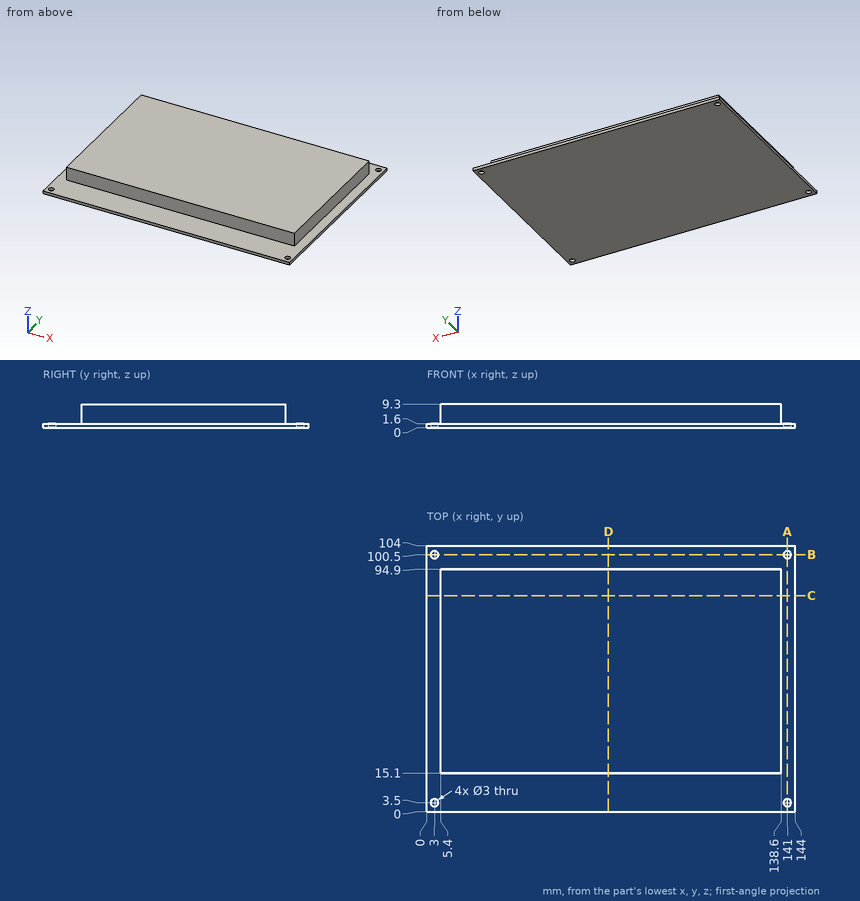
Geometry check sheet. Reference: drawing and pictorial views, mm from the part's lowest x, y, z. Round coordinates to 2 decimals unless told otherwise and drop trailing zeros. Loops run counter-clockwise (first coordinate to the right, second up) from the corner with the lowest first, then second, coordinate; pieces in that order, holes last. Notation, with made-up numbers: (6, 16) - (16, 16) arc R6 ccw to (16, 21) - close; hole circle Ø11 at (36, -31.75). An arc over 180 degrees is marked (long way). One line per question, with ' | ' between items. Start each with the question number.
1. Cross-section at A-A on x = 141. Record the cut outline in (y, z), then the cut area to 3 significant figures.
2. Depth check by flat-ended pin: pin 1 (2.5 mm diameter, centred on y = 43, z = 6, fed in from +X); pin 2 (4 mm diameter, centred on y = 47.5, z = 5.5, fed in from -X); pin 3 (5 mm diameter, centred on x = 141, y = 3.5, fed in from +Z). Enter the tip coordinate at first touch or a pass-through.
3. Cross-section at C-C on y = 84.5. Record the cut outline in (x, z).
4. Cross-section at B-B on y = 100.5. Record the cut outline in (x, z), then the cut area to 3 significant figures.
5. Scan lines: line 1 (X direction, y = 100.5, z = 0.8); line 2 (Y direction, x = 3, z = 1.1); line 3 (Z direction, x = 54, y = 10). Record each from-to range of solid material in increasing order. Write a range as [from, to].
6. Cross-section at D-D on x = 71. Record the cut outline in (y, z), then the cut area to 3 significant figures.
Taken from the geometry:
1) outline: (0, 0) - (2, 0) - (2, 1.6) - (0, 1.6) - close; (5, 0) - (99, 0) - (99, 1.6) - (5, 1.6) - close; (102, 0) - (104, 0) - (104, 1.6) - (102, 1.6) - close | area: 157 mm²
2) pin 1: x = 138.6 | pin 2: x = 5.4 | pin 3: z = 1.6
3) outline: (0, 0) - (144, 0) - (144, 1.6) - (138.6, 1.6) - (138.6, 9.3) - (5.4, 9.3) - (5.4, 1.6) - (0, 1.6) - close
4) outline: (0, 0) - (1.5, 0) - (1.5, 1.6) - (0, 1.6) - close; (4.5, 0) - (139.5, 0) - (139.5, 1.6) - (4.5, 1.6) - close; (142.5, 0) - (144, 0) - (144, 1.6) - (142.5, 1.6) - close | area: 221 mm²
5) line 1: [0, 1.5], [4.5, 139.5], [142.5, 144] | line 2: [0, 2], [5, 99], [102, 104] | line 3: [0, 1.6]
6) outline: (0, 0) - (104, 0) - (104, 1.6) - (94.9, 1.6) - (94.9, 9.3) - (15.1, 9.3) - (15.1, 1.6) - (0, 1.6) - close | area: 781 mm²
